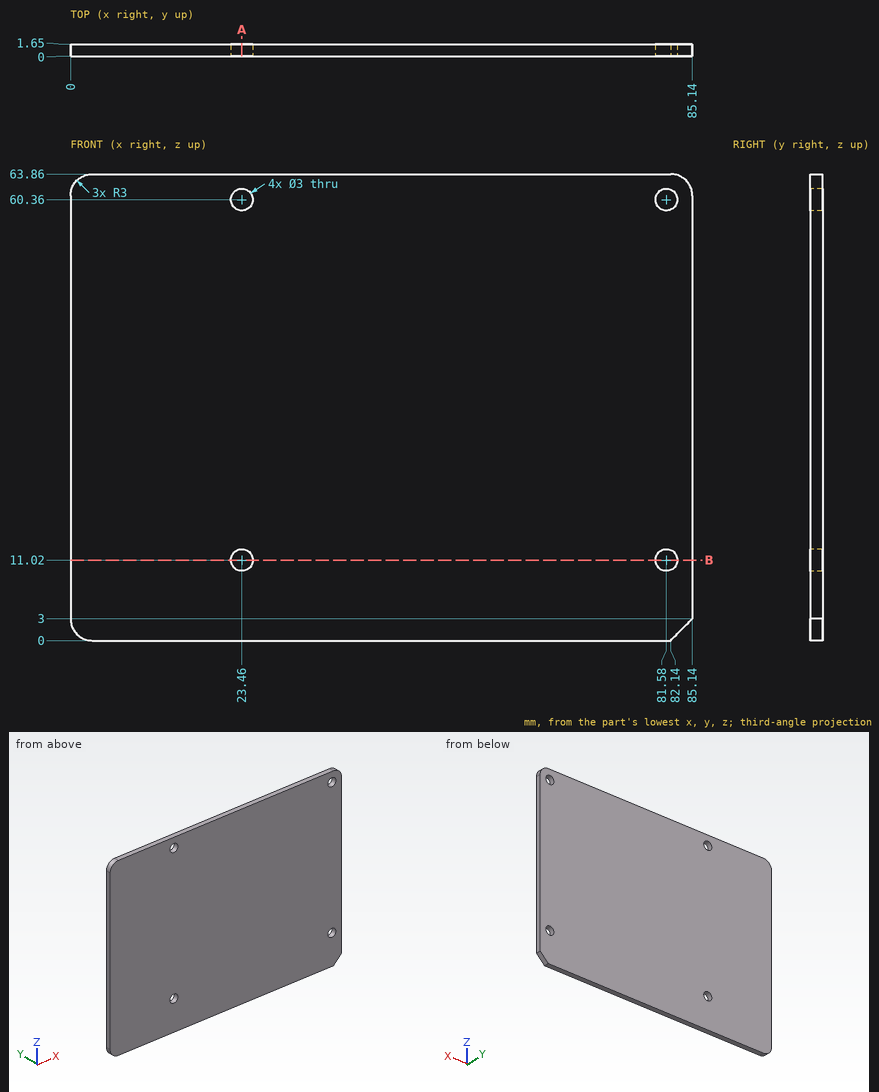
Geometry check sheet. Reference: drawing and pictorial views, mm from the part's lowest x, y, z. Coordinates: 2 decimals unless noted, no trailing zeros. Write each loop counter-clockwise with the first axis right and the second up, starting at its lowest first coordinate (ties: lowest second). Pieces come first, ordered by that corner, then holes. Notation, with made-up numbers: M 55.25,0.5 L 109.25,0.5 A25 ccw 109.25,22.5 Z; hole C -37.75,78.25 d7. An arc over 180 degrees is marked long. Write item = value, one per line. Start each with the question number.
1. Sectioned sample at A-A (x = 23.46). Record the cut outline in (y, z), then the cut area to 3 significant figures.
2. Go/stop test with a flat-tipped pin: pin 1 (2.5 mm diameter, centred on x = 81.58, z = 11.02, fed in from +Y). Record where the tip stops, or that it passes through.
3. Sectioned sample at B-B (z = 11.02). Record the cut outline in (x, y), then the cut area to 3 significant figures.
4. Thickness scan on probe 1 along X at (y, z) = (1.35, 60.36); probe 2 along Z at (x, y) = (23.46, 0.65); probe 3 along Z at (x, y) = (23, 1.1). Record the ranges inside material, lowest first.
The answers:
q1.outline = M 0,0 L 1.65,0 L 1.65,9.52 L 0,9.52 Z; M 0,12.52 L 1.65,12.52 L 1.65,58.86 L 0,58.86 Z; M 0,61.86 L 1.65,61.86 L 1.65,63.86 L 0,63.86 Z
q1.area = 95.5 mm²
q2.pin_1 = through
q3.outline = M 0,0 L 21.96,0 L 21.96,1.65 L 0,1.65 Z; M 24.96,0 L 80.08,0 L 80.08,1.65 L 24.96,1.65 Z; M 83.08,0 L 85.14,0 L 85.14,1.65 L 83.08,1.65 Z
q3.area = 131 mm²
q4.probe_1 = 0 to 21.96, 24.96 to 80.08, 83.08 to 85.14
q4.probe_2 = 0 to 9.52, 12.52 to 58.86, 61.86 to 63.86
q4.probe_3 = 0 to 9.59, 12.45 to 58.93, 61.79 to 63.86
